Part model, mm, in its own coordinate system. A direction names the side the tool comes from. Round coordinates to 2 decimals unless told otherwise and drop trailing zeros. Write each loop counter-clockwise with the first axis right and the second up, starting at its lowest first coordinate (ties: lowest second). Pieces come first, ordered by that corner, then holes. Notation, with made-up numbers: M -23,24.5 L 36,24.5 A19 ccw 36,42.5 Z; hole C 50.5,29.5 d10. An arc over 180 degrees is marked long. One line per question, with ' | ' between items. Start each with the question number.
1) Saw through at B-B (y = 18). List the corners of the cut face in (x, z).
2) Saw through at A-A (y = -6). List the corners of the cut face in (x, z).
3) Mould opens along Y. For faces 1 (the face through (1.5, 15, 0)), 2 (the face through (2, -2, 14)), 3 (the face through (-3, -10, 14)), 4 (the face through (-2.48, -7.19, 13.01)) say: pulls with the +Y half, pulls with the -Y half, needs draft (parallel to the pull), parting line crosses it, or undercut.
4) Saw through at C-C (x = -7.25). List the corners of the cut face in (y, z), plus the area to 3 significant figures.
5) Wall check: probe 1 along X at (y, z) = (-7.5, 10); probe 2 along Z at (x, y) = (1.2, -6); probe 3 along Z at (x, y) = (-2.25, -5). Give the ranges that are in metal, low to high. Write a range as [from, to].
6) Saw through at D-D (z = 2.5). List the corners of the cut face in (x, y), plus the area to 3 significant figures.
7) Tool access for faces 5 (the face through (4, -6, 11)), 6 (the face through (0, 0, -2)), 7 (the face through (-3, -6, 17.748)), 8 (the face through (1, -6, 10)), 9 (the face through (3, -6, 11.174)): list every direction of +Z, -Z, +X, -X, +Y, -Y with a clear straight run to the whole face (end or side of a thin tool).
8) Drop flat-ended pins along their axis: pin 1 Ø1 at (x, z) = (2.5, 10.5) entering from +Y; pin 2 Ø8 at (y, z) = (2, 8.5) entering from +X; pin 3 Ø9.5 at (x, z) = (0, 0) entering from -Y. Give the stop position or say it passes through.
```python
from build123d import *
from build123d import SkipClean  # not in build123d's __all__

# Parameters (mm, degrees)
F1_DEPTH  = 12
F0_W      = 3
F0_H      = 2.5
F2_DEPTH  = 10
F3_DEPTH  = 2
F5_R      = 1.5
F6_DEPTH  = 25
F7_DEPTH  = 2.3
F9_DEPTH  = 0.5
F11_ANGLE = 180
F12_DEPTH = 1.5


with BuildPart() as f1:
    # F0 (on Front) → F1 (new body)
    with BuildSketch(Plane.XZ):
        with BuildLine():
            Line((-4, 9.3285851017), (-1, 9.3285851017))
            Line((-1, 9.3285851017), (-1, 10.1006187929))
            ThreePointArc((-1, 10.1006187929), (-2.529626258, 9.8297248687), (-4, 9.3285851017))
        make_face()
        with BuildLine():
            Line((1, 10.1006187929), (1, 9.3285851017))
            Line((1, 9.3285851017), (4, 9.3285851017))
            ThreePointArc((4, 9.3285851017), (2.529626258, 9.8297248687), (1, 10.1006187929))
        make_face()
        with BuildLine():
            ThreePointArc((1, 5.0519798099), (3.9794786091, 3.2689830223), (5.15, 0))
            ThreePointArc((5.15, 0), (-3.2689830223, -3.9794786091), (-1, 5.0519798099))
            Line((-1, 5.0519798099), (-1, 9.3285851017))
            Line((-1, 9.3285851017), (-4, 9.3285851017))
            ThreePointArc((-4, 9.3285851017), (-5.5867029633, -8.474151875), (10.15, 0))
            ThreePointArc((10.15, 0), (8.474151875, 5.5867029633), (4, 9.3285851017))
            Line((4, 9.3285851017), (1, 9.3285851017))
            Line((1, 9.3285851017), (1, 5.0519798099))
        make_face()
    extrude(amount=F1_DEPTH)

    # F0 (on Front) → F2 (join)
    with BuildSketch(Plane.XZ):
        with BuildLine():
            ThreePointArc((-4, 9.3285851017), (-2.529626258, 9.8297248687), (-1, 10.1006187929))
            Line((-1, 10.1006187929), (-1, 15.2480201901))
            Line((-1, 15.2480201901), (-4, 15.2480201901))
            Line((-4, 15.2480201901), (-4, 9.3285851017))
        make_face()
        with BuildLine():
            Line((1, 15.2480201901), (1, 10.1006187929))
            ThreePointArc((1, 10.1006187929), (2.529626258, 9.8297248687), (4, 9.3285851017))
            Line((4, 9.3285851017), (4, 15.2480201901))
            Line((4, 15.2480201901), (1, 15.2480201901))
        make_face()
        with Locations((-2.5, 16.4980201901)):
            Rectangle(F0_W, F0_H)
        with Locations((2.5, 16.4980201901)):
            Rectangle(F0_W, F0_H)
    extrude(amount=F2_DEPTH)

    # F0 (on Front) → F3 (cut)
    with BuildSketch(Plane.XZ):
        with BuildLine():
            ThreePointArc((-4, 9.3285851017), (-2.529626258, 9.8297248687), (-1, 10.1006187929))
            Line((-1, 10.1006187929), (-1, 15.2480201901))
            Line((-1, 15.2480201901), (-4, 15.2480201901))
            Line((-4, 15.2480201901), (-4, 9.3285851017))
        make_face()
        with BuildLine():
            Line((1, 15.2480201901), (1, 10.1006187929))
            ThreePointArc((1, 10.1006187929), (2.529626258, 9.8297248687), (4, 9.3285851017))
            Line((4, 9.3285851017), (4, 15.2480201901))
            Line((4, 15.2480201901), (1, 15.2480201901))
        make_face()
        with Locations((-2.5, 16.4980201901)):
            Rectangle(F0_W, F0_H)
        with Locations((2.5, 16.4980201901)):
            Rectangle(F0_W, F0_H)
    with SkipClean():  # cleaning this boolean's faces spoils the solid; the shape is the same uncleaned
        extrude(amount=F3_DEPTH, mode=Mode.SUBTRACT)

    # F5 (on face) → F6 (cut)
    with BuildSketch(Plane.YZ.offset(4)):
        with Locations((-6, 13.9243194915)):
            Circle(F5_R)
    extrude(amount=-F6_DEPTH, mode=Mode.SUBTRACT)

    # F5 (on face) → F7 (cut)
    with BuildSketch(Plane.YZ.offset(4)):
        Polygon((-4.4122867597, 16.6743194915), (-7.5877132403, 16.6743194915), (-9.1754264805, 13.9243194915), (-7.5877132403, 11.1743194915), (-4.4122867597, 11.1743194915), (-2.8245735195, 13.9243194915), align=None)
        with Locations((-6, 13.9243194915)):
            Circle(F5_R, mode=Mode.SUBTRACT)
    extrude(amount=-F7_DEPTH, mode=Mode.SUBTRACT)

    # F8 (on face) → F9 (join)
    with BuildSketch(Plane.XZ):
        with BuildLine():
            Line((10.15, 0), (5.15, 0))
            ThreePointArc((5.15, 0), (0, -5.15), (-5.15, 0))
            Line((-5.15, 0), (-10.15, 0))
            ThreePointArc((-10.15, 0), (0, -10.15), (10.15, 0))
        make_face()
        with BuildLine():
            ThreePointArc((-5.15, 0), (0, -5.15), (5.15, 0))
            Line((5.15, 0), (-5.15, 0))
        make_face()
    extrude(amount=-F9_DEPTH)

    # F9_face (on face) → F11 (revolve)
    with BuildSketch(Plane(origin=(0, 0.5, -4.307793793), x_dir=(1, 0, 0), z_dir=(0, 1, 0))):
        with BuildLine():
            Line((-10.15, -4.307793793), (10.15, -4.307793793))
            ThreePointArc((10.15, -4.307793793), (0, 5.842206207), (-10.15, -4.307793793))
        make_face()
    revolve(axis=Axis((0, 0.5, 0), (1, 0, 0)), revolution_arc=F11_ANGLE)

    # F10 (on Right) → F12 (join, symmetric)
    with BuildSketch(Plane.YZ):
        with BuildLine():
            ThreePointArc((17, 4.5), (13.8180194847, 3.1819805153), (12.5, 0))
            Line((12.5, 0), (15.5, 0))
            ThreePointArc((15.5, 0), (15.9393398282, 1.0606601718), (17, 1.5))
            Line((17, 1.5), (17, 4.5))
        make_face()
        with BuildLine():
            ThreePointArc((9.0979393271, 4.5), (9.8834858266, 2.3106726109), (10.15, 0))
            Line((10.15, 0), (12.5, 0))
            ThreePointArc((12.5, 0), (13.8180194847, 3.1819805153), (17, 4.5))
            Line((17, 4.5), (9.0979393271, 4.5))
        make_face()
        with BuildLine():
            Line((12.5, 0), (10.15, 0))
            ThreePointArc((10.15, 0), (9.8834858266, -2.3106726109), (9.0979393271, -4.5))
            Line((9.0979393271, -4.5), (17, -4.5))
            ThreePointArc((17, -4.5), (13.8180194847, -3.1819805153), (12.5, 0))
        make_face()
        with BuildLine():
            Line((15.5, 0), (12.5, 0))
            ThreePointArc((12.5, 0), (13.8180194847, -3.1819805153), (17, -4.5))
            ThreePointArc((17, -4.5), (20.1819805153, -3.1819805153), (21.5, 0))
            ThreePointArc((21.5, 0), (20.1819805153, 3.1819805153), (17, 4.5))
            Line((17, 4.5), (17, 1.5))
            ThreePointArc((17, 1.5), (18.0606601718, 1.0606601718), (18.5, 0))
            ThreePointArc((18.5, 0), (17, -1.5), (15.5, 0))
        make_face()
    extrude(amount=F12_DEPTH, both=True)


solid = f1.part
```
Answer key:
1) outline: M -1.5,-4.39 L 1.5,-4.39 L 1.5,-1.12 L -1.5,-1.12 Z; M -1.5,1.12 L 1.5,1.12 L 1.5,4.39 L -1.5,4.39 Z
2) outline: M -4,9.33 A10.15 ccw long 4,9.33 L 4,11.17 L 1.7,11.17 L 1.7,12.42 L 1,12.42 L 1,5.05 A5.15 cw long -1,5.05 L -1,12.42 L -4,12.42 Z; M -4,15.42 L -1,15.42 L -1,17.75 L -4,17.75 Z; M 1,15.42 L 1.7,15.42 L 1.7,16.67 L 4,16.67 L 4,17.75 L 1,17.75 Z
3) face 1: needs draft | face 2: pulls with the +Y half | face 3: pulls with the -Y half | face 4: undercut
4) outline: M -12,-7.1 L 0.5,-7.1 A7.1 ccw 0.5,7.1 L 0.5,0 L 0,0 L 0,7.1 L -12,7.1 Z | area: 253 mm2
5) probe 1: x = [-4, -1], [1, 4] | probe 2: z = [-10.08, -5.01], [5.01, 12.42], [15.42, 17.75] | probe 3: z = [-9.9, -4.63], [4.63, 12.81], [15.04, 17.75]
6) outline: M -9.84,-12 L -4.5,-12 L -4.5,0 L -9.84,0 Z; M -9.84,0.5 L 9.84,0.5 A9.84 ccw 1.5,10.22 L 1.5,20.74 L -1.5,20.74 L -1.5,10.22 A9.84 ccw Z; M 4.5,-12 L 9.84,-12 L 9.84,0 L 4.5,0 Z | area: 311 mm2
7) face 5: +Z, +X, +Y, -Y | face 6: -Y | face 7: +Z, +X, -X, +Y, -Y | face 8: +Z, -Y | face 9: +X
8) pin 1: stops at y = -2 | pin 2: stops at x = 9.03 | pin 3: stops at y = 0
